Check sheet for the modelled part. Datum: model origin and axes. Units: mm. Face numbers are marked on the shaded views. A direction names the side the tool comes from. Coordinates: 2 decimals unless noted, no trailing zeros. Loops run counter-clockwise (first coordinate to the right, second up) from the corner with the lowest first, then second, coordinate; pieces in that order, holes last. Notation, with made-up numbers: (27, 82.25) - (46, 82.25) arc R18 ccw to (46, 96.25) - close; hole circle Ø6 at (57.25, 35). An arc over 180 degrees is marked (long way). Write each question's results on one line, items separated by ' | '. Start each with the question number.
1. Thickness scan on line 1 (Y direction, x = 0, z = 2.3); line 2 (Y direction, x = 0, z = 1.3); line 3 (Z direction, x = 2.75, y = -0.5). Record the ranges inside material, lowest first. Write a range as [from, to].
2. Draft check along X on the marked faces 4, 5 and 6. Enter one of: released by +X, released by -X, zero draft, split by the parting line, or undercut.
3. Cross-section at A-A (y = 0). Record the cut outline in (x, z), and give its area (3 significant figures).
4. Tool access check on the marked faces 1, 2 and 3. Record the directions out of +Z, -Z, +X, -X, +Y, -Y that give a thin tool (end or side, any length) a straight path to the whole face; none if there is none.
5. Gauge pin test, flat ends, axial feed: P1, Ø1, axis at y = -2, z = 1.5, coming from the +X side; P2, Ø1, axis at x = 2.5, y = -1.5, coming from the -Z side. Record the tip position at first contact, or that the pin passes through.
6. Cross-section at D-D (y = 2.25). Record the cut outline in (x, z).
7. Cross-section at C-C (z = 2.2). Record the cut outline in (x, y).
Autodesk Inventor part; units mm, degrees
ref_plane "Work Plane1" through (0, 0, 1.25) normal (0, 0, 1) x (1, 0, 0)
ref_plane "YZ Plane" through (0, 0, 0) normal (1, 0, 0) x (0, 1, 0)
ref_plane "XZ Plane" through (0, 0, 0) normal (0, 1, 0) x (-1, 0, 0)
sketch "Sketch1" plane through (0, 0, 0) normal (0, 0, 1) x (1, 0, 0)
  circle A0 centre (0, 0) radius 3.5
  dimension "d0" = 7
extrude "Extrusion1" add sketch "Sketch1" along normal blind 2.5
hole "Hole1" at (0, 0, 2.5) direction (0, 0, -1) diameter 4 end through all
sketch "Sketch2" plane through (0, 0, 2.5) normal (0, 0, 1) x (1, 0, 0)
  circle A0 centre (0, 0) radius 3
  circle A1 centre (0, 0) radius 2.5
  dimension "d12" = 6
  dimension "d13" = 5
extrude "Extrusion2" cut sketch "Sketch2" against normal blind 0.5
ref_plane "Work Plane1" through (0, 0, 1.25) normal (0, 0, 1) x (1, 0, 0)
mirror "Mirror1" about plane through (0, 0, 1.25) normal (0, 0, 1) of "Extrusion2"
properties part number "bearing_4x7x2.5_74" material "Stainless Steel"
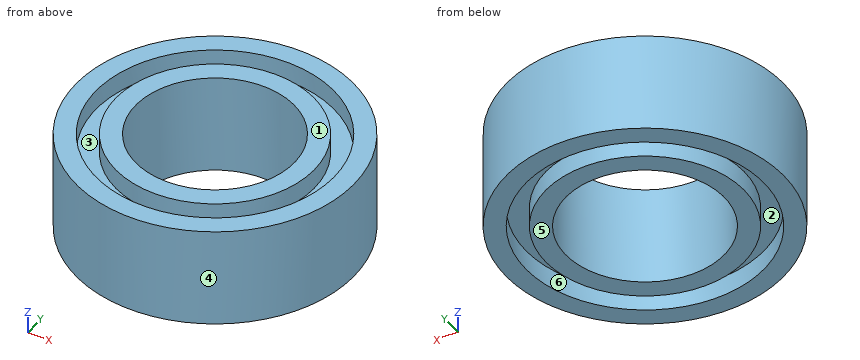
Established:
1) line 1: [-3.5, -3], [-2.5, -2], [2, 2.5], [3, 3.5] | line 2: [-3.5, -2], [2, 3.5] | line 3: [0.5, 2]
2) face 4: split by the parting line | face 5: zero draft | face 6: undercut
3) outline: (-3.5, 0) - (-3, 0) - (-3, 0.5) - (-2.5, 0.5) - (-2.5, 0) - (-2, 0) - (-2, 2.5) - (-2.5, 2.5) - (-2.5, 2) - (-3, 2) - (-3, 2.5) - (-3.5, 2.5) - close; (2, 0) - (2.5, 0) - (2.5, 0.5) - (3, 0.5) - (3, 0) - (3.5, 0) - (3.5, 2.5) - (3, 2.5) - (3, 2) - (2.5, 2) - (2.5, 2.5) - (2, 2.5) - close | area: 6.50 mm^2
4) face 1: +Z, +X, -X, +Y, -Y | face 2: -Z | face 3: +Z
5) P1: x = 3.16 | P2: z = 0
6) outline: (-2.68, 0) - (-1.98, 0) - (-1.98, 0.5) - (-1.09, 0.5) - (-1.09, 0) - (1.09, 0) - (1.09, 0.5) - (1.98, 0.5) - (1.98, 0) - (2.68, 0) - (2.68, 2.5) - (1.98, 2.5) - (1.98, 2) - (1.09, 2) - (1.09, 2.5) - (-1.09, 2.5) - (-1.09, 2) - (-1.98, 2) - (-1.98, 2.5) - (-2.68, 2.5) - close
7) outline: circle Ø7 at (0, 0); circle Ø5 at (0, 0); hole circle Ø6 at (0, 0); hole circle Ø4 at (0, 0)
